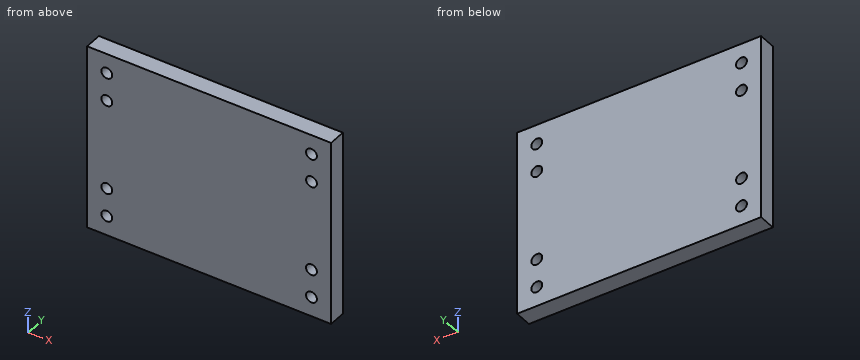
from build123d import *

# Parameters (mm, degrees)
SKETCH1_W                       = 22.4
SKETCH1_H                       = 17.1
MAIN_BODY_DEPTH                 = 1.6
SKETCH2_R                       = 0.5
SOLDERED_CONNECTION_HOLES_DEPTH = 15.181061314
MIRROR2_COPY_1_SKETCH_R         = 0.5
MIRROR2_COPY_1_DEPTH            = 15.181061314


with BuildPart() as part:
    # Sketch1 → MAIN BODY (new body)
    with BuildSketch(Plane(origin=(0, 0, 0), x_dir=(1, 0, 0), z_dir=(0, 1, 0))):
        Rectangle(SKETCH1_W, SKETCH1_H)
    extrude(amount=MAIN_BODY_DEPTH)

    # Sketch2 → SOLDERED CONNECTION HOLES (cut, through all)
    with BuildSketch(Plane(origin=(0, 1.6, 0), x_dir=(1, 0, 0), z_dir=(0, 1, 0))):
        with Locations(Location((-9.4, 6.75, 0), (0, 0, 270))):
            Circle(SKETCH2_R)
        with Locations(Location((-9.4, 4.15, 0), (0, 0, 270))):
            Circle(SKETCH2_R)
    soldered_connection_holes = extrude(amount=-SOLDERED_CONNECTION_HOLES_DEPTH, mode=Mode.SUBTRACT)

    # Mirror1: SOLDERED CONNECTION HOLES across plane
    add(soldered_connection_holes.mirror(Plane(origin=(0, 0, 0), x_dir=(0, 0, 1), z_dir=(1, 0, 0))), mode=Mode.SUBTRACT)

    # Mirror2: SOLDERED CONNECTION HOLES across plane
    add(soldered_connection_holes.mirror(Plane.XY), mode=Mode.SUBTRACT)

    # Mirror2 copy 1 sketch → Mirror2 copy 1 (cut, through all)
    with BuildSketch(Plane(origin=(0, 1.6, 0), x_dir=(-1, 0, 0), z_dir=(0, 1, 0))):
        with Locations(Location((-9.4, 6.75, 0), (0, 0, 270))):
            Circle(MIRROR2_COPY_1_SKETCH_R)
        with Locations(Location((-9.4, 4.15, 0), (0, 0, 270))):
            Circle(MIRROR2_COPY_1_SKETCH_R)
    extrude(amount=-MIRROR2_COPY_1_DEPTH, mode=Mode.SUBTRACT)


solid = part.part
Could you check a few things on this model? Use its own coordinates, in mm. Coordinates: 2 decimals unless noted, no trailing zeros. Write each loop counter-clockwise with the first axis right and the second up, starting at its lowest first coordinate (ties: lowest second). Pieces come first, ordered by that corner, then holes. Notation, with made-up numbers: (-32.5, 59.5) - (15.5, 59.5) arc R31 cw to (15.5, 91.5) - close; hole circle Ø4 at (68.5, 66.5). An arc over 180 degrees is marked (long way). Put each result on its own line as item: value. Start each with the question number.
Q1. I want a section at B-B on x = 9.4. Write out the boundary of the cut face in (y, z), plus the area to 3 significant figures.
Q2. I want a section at C-C on y = 1.1. Count the separate pieces of the cut face and the enclosed holes in it, plus the area to 3 significant figures.
Q3. Please list where these lines run through material, in increasing order: L1, parallel to X at y = 0.8, z = -6.75; L2, parallel to Z at x = 9.4, y = 0.3; L3, parallel to X at y = 1.35, z = -4.5.
Q4. I want a section at A-A on z = -4.15. Write out the boundary of the cut face in (x, y), plus the area to 3 significant figures.
Checks:
1. outline: (0, -8.55) - (1.6, -8.55) - (1.6, -7.25) - (0, -7.25) - close; (0, -6.25) - (1.6, -6.25) - (1.6, -4.65) - (0, -4.65) - close; (0, -3.65) - (1.6, -3.65) - (1.6, 3.65) - (0, 3.65) - close; (0, 4.65) - (1.6, 4.65) - (1.6, 6.25) - (0, 6.25) - close; (0, 7.25) - (1.6, 7.25) - (1.6, 8.55) - (0, 8.55) - close
1. area: 21.0 mm²
2. separate pieces: 1
2. enclosed holes: 8
2. area: 377 mm²
3. L1: -11.2 to -9.9, -8.9 to 8.9, 9.9 to 11.2
3. L2: -8.55 to -7.25, -6.25 to -4.65, -3.65 to 3.65, 4.65 to 6.25, 7.25 to 8.55
3. L3: -11.2 to -9.76, -9.04 to 9.04, 9.76 to 11.2
4. outline: (-11.2, 0) - (-9.9, 0) - (-9.9, 1.6) - (-11.2, 1.6) - close; (-8.9, 0) - (8.9, 0) - (8.9, 1.6) - (-8.9, 1.6) - close; (9.9, 0) - (11.2, 0) - (11.2, 1.6) - (9.9, 1.6) - close
4. area: 32.6 mm²
